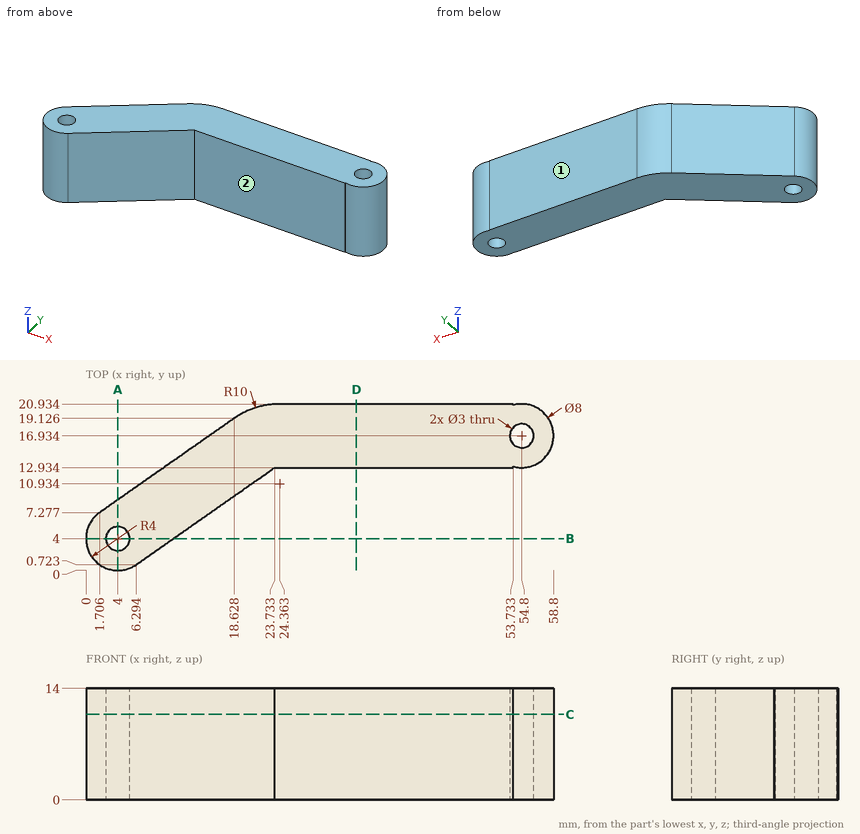
Source: three-view drawing plus pictorial views. Frame: mm from the lowest corner of the part. A direction names the side the tool comes from. Round coordinates to 2 decimals unless told otherwise and drop trailing zeros. Loops run counter-clockwise (first coordinate to the right, second up) from the corner with the lowest first, then second, coordinate; pieces in that order, holes last.
Q1. Material intervals for L1, parallel to Y at x = 36, z = 7.25; L2, parallel to X at y = 4, z = 6.25 (1 decimal); L3, parallel to Y at x = 4, z = 9.25 (1 decimal), sorted ascending.
Q2. Section A-A on x = 4. Return loops of the section in (y, z).
Q3. Section D-D on x = 34. Return loops of the section in (y, z), plus the area to 3 significant figures.
Q4. Pin query (flat end, axial travel): P1, Ø4, axis at y = 6.5, z = 7, coming from the -X side; P2, Ø7, axis at x = 36.5, z = 7.5, coming from the -Y side. Return the tip coordinate at first contact, or that it passes through.
Q5. Section C-C on z = 10.75. State how many separate pieces and enclosed holes the cut face has, plus the area to 3 significant figures.
Q6. Section B-B on y = 4. Return loops of the section in (x, z), plus the area to 3 significant figures.
Q7. Access query for the marked faces 1 and 2. Directions: +Z, -Z, +X, -X, +Y, -Y. A direction counts if a zero-diameter tool reaches every point of the face in a straight line with its end or side. Return the directions, or none.
Evaluation:
1. L1: y = 12.93 to 20.93
1. L2: x = 0 to 2.5, 5.5 to 11
1. L3: y = 0 to 2.5, 5.5 to 8.9
2. outline: (0, 0) - (2.5, 0) - (2.5, 14) - (0, 14) - close; (5.5, 0) - (8.88, 0) - (8.88, 14) - (5.5, 14) - close
3. outline: (12.93, 0) - (20.93, 0) - (20.93, 14) - (12.93, 14) - close
3. area: 112 mm2
4. P1: stops at x = 0.03
4. P2: stops at y = 12.93
5. separate pieces: 1
5. enclosed holes: 2
5. area: 474 mm2
6. outline: (0, 0) - (2.5, 0) - (2.5, 14) - (0, 14) - close; (5.5, 0) - (10.97, 0) - (10.97, 14) - (5.5, 14) - close
6. area: 112 mm2
7. face 1: +Z, -Z, +X, -X, +Y
7. face 2: +Z, -Z, +X, -Y
